Source: CAD feature listing. Evaluate the final solid. Frame: model axes, mm. Face numbers are marked on the shaded views. A direction names the side the tool comes from. Round coordinates to 2 decimals unless told otherwise and drop trailing zeros. Write each loop counter-clockwise with the first axis right and the second up, starting at its lowest first coordinate (ties: lowest second). Pieces come first, ordered by that corner, then holes.
from build123d import *

# Parameters (mm, degrees)
F3_DEPTH      = 5
F3_DEPTH_BACK = 5


with BuildPart() as f1:
    # F0 (on Front) → F1 (revolve)
    with BuildSketch(Plane.XZ):
        with BuildLine():
            Line((0.25, 7), (0.25, 0))
            Line((0.25, 0), (6.5, 0))
            Line((6.5, 0), (6.5, 1))
            Line((6.5, 1), (4.25, 1))
            Line((4.25, 1), (2.75, 2.5))
            ThreePointArc((2.75, 2.5), (3.1793149932, 4.527027027), (2.75, 6.5540540541))
            ThreePointArc((2.75, 6.5540540541), (2.4733345666, 6.8787052332), (2.064397249, 7))
            Line((2.064397249, 7), (0.25, 7))
        make_face()
    revolve(axis=Axis((0, 0, 4.4036353938), (0, 0, 1)))


with BuildPart() as f3:
    # F2 (on Front) → F3 (new body, two sides)
    with BuildSketch(Plane.XZ) as f3_sk:
        with BuildLine():
            Line((4.25, 7.1200682409), (3.25, 7.1200682409))
            ThreePointArc((3.25, 7.1200682409), (2.5801270189, 4.6200682409), (3.25, 2.1200682409))
            Line((3.25, 2.1200682409), (4.25, 2.1200682409))
            Line((4.25, 2.1200682409), (4.25, 7.1200682409))
        make_face()
    extrude(amount=F3_DEPTH)
    extrude(f3_sk.sketch, amount=-F3_DEPTH_BACK)


with BuildPart() as f4_1:
    # F4: instance of F3
    add(f3.part.mirror(Plane.YZ))


with BuildPart() as f1_1:
    add(f1.part)

    # F5: cut F3, F4_1
    add(f3.part, mode=Mode.SUBTRACT)
    add(f4_1.part, mode=Mode.SUBTRACT)


solid = f1_1.part
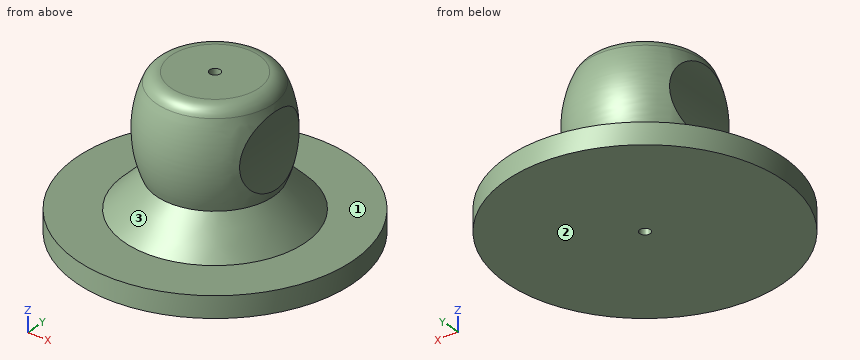
1) Material intervals for line 1 (Y direction, x = 0, z = 4.5); line 2 (Z direction, x = 0.75, y = 5.75); line 3 (Y direction, x = 0, z = 2.75), sorted ascending.
Taken from the geometry:
line 1: y = -3.18 to -0.25, 0.25 to 3.18
line 2: z = 0 to 1
line 3: y = -2.85 to -0.25, 0.25 to 2.85
2) Section query A-A on x = -4.75. Return the cut outline in (y, z), then the cut area to 3 significant figures.
Taken from the geometry:
outline: (-4.44, 0) - (4.44, 0) - (4.44, 1) - (-4.44, 1) - close
area: 8.87 mm2
3) Contact query for flat-ended pins moving along their axis: P1, Ø1.5, axis at y = 3.5, z = 6, coming from the +X side; P2, Ø2, axis at x = -0.5, z = 5, coming from the +Y side; P3, Ø2, axis at y = 1, z = 4.5, coming from the +X side. Output: stop coordinate, or through.
Taken from the geometry:
P1: stops at x = 1.17
P2: stops at y = 3.18
P3: stops at x = 2.71
4) Reachability of the marked faces 1, 2 and 3 from +Z, -Z, +X, -X, +Y, -Y: full face, straight path, thin tool, end or side. Return the list, or none.
Taken from the geometry:
face 1: +Z
face 2: -Z, +X, -X, +Y, -Y
face 3: none
